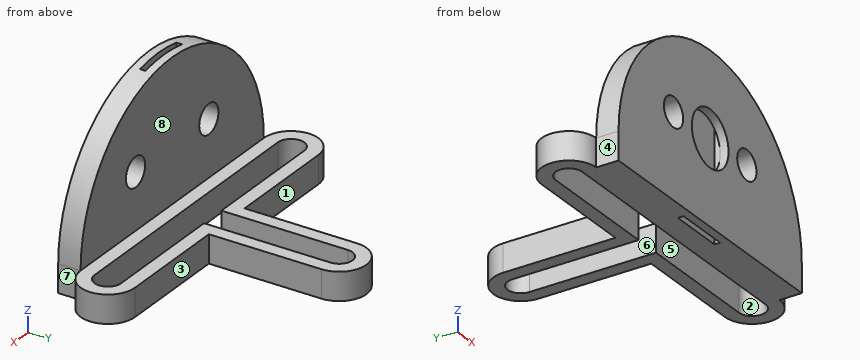
```python
from build123d import *

# Parameters (mm, degrees)
SKETCH1_W           = 100
SKETCH1_H           = 8
BOSS_EXTRUDE1_DEPTH = 10
BOSS_EXTRUDE2_DEPTH = 8
SKETCH3_R           = 5.25
CUT_EXTRUDE1_DEPTH  = 105.404561682
SKETCH4_W           = 20
SKETCH4_H           = 2
CUT_EXTRUDE2_DEPTH  = 104.634574347
SKETCH5_R           = 10
CUT_EXTRUDE3_DEPTH  = 3


with BuildPart() as part:
    # Sketch1 → Boss-Extrude1 (new body)
    # profile 1 of 2: a face of its own
    with BuildSketch(Plane.XY):
        with BuildLine():
            ThreePointArc((-9.75, 50), (0, 59.75), (9.75, 50))
            Line((9.75, 50), (9.75, 9.75))
            Line((9.75, 9.75), (50, 9.75))
            ThreePointArc((50, 9.75), (59.75, 0), (50, -9.75))
            Line((50, -9.75), (-50, -9.75))
            ThreePointArc((-50, -9.75), (-59.75, 0), (-50, 9.75))
            Line((-50, 9.75), (-9.75, 9.75))
            Line((-9.75, 9.75), (-9.75, 50))
        make_face()
        with BuildLine():
            Line((4.75, 4.75), (50, 4.75))
            ThreePointArc((50, 4.75), (54.75, 0), (50, -4.75))
            Line((50, -4.75), (-50, -4.75))
            ThreePointArc((-50, -4.75), (-54.75, 0), (-50, 4.75))
            Line((-50, 4.75), (-4.75, 4.75))
            Line((-4.75, 4.75), (-4.75, 50))
            ThreePointArc((-4.75, 50), (0, 54.75), (4.75, 50))
            Line((4.75, 50), (4.75, 4.75))
        make_face(mode=Mode.SUBTRACT)
    # profile 2 of 2: a face of its own
    with BuildSketch(Plane.XY):
        with Locations((0, -13.75)):
            Rectangle(SKETCH1_W, SKETCH1_H)
    extrude(amount=-BOSS_EXTRUDE1_DEPTH)

    # Sketch2 → Boss-Extrude2 (add)
    with BuildSketch(Plane.XZ.offset(17.75)):
        with BuildLine():
            Line((-50, 0), (50, 0))
            ThreePointArc((50, 0), (0, 50), (-50, 0))
        make_face()
    extrude(amount=-BOSS_EXTRUDE2_DEPTH)

    # Sketch3 → Cut-Extrude1 (cut, through all)
    with BuildSketch(Plane(origin=(0, -9.75, 0), x_dir=(1, 0, 0), z_dir=(0, 1, 0))):
        with Locations(Location((20, -20, 0), (0, 0, 270))):
            Circle(SKETCH3_R)
        with Locations(Location((-20, -20, 0), (0, 0, 270))):
            Circle(SKETCH3_R)
    extrude(amount=-CUT_EXTRUDE1_DEPTH, mode=Mode.SUBTRACT)

    # Sketch4 → Cut-Extrude2 (cut, through all)
    with BuildSketch(Plane(origin=(0, 0, -10), x_dir=(-1, 0, 0), z_dir=(0, 0, -1))):
        with Locations((0, -13.75)):
            Rectangle(SKETCH4_W, SKETCH4_H)
    extrude(amount=-CUT_EXTRUDE2_DEPTH, mode=Mode.SUBTRACT)

    # Sketch5 → Cut-Extrude3 (cut)
    with BuildSketch(Plane.XZ.offset(17.75)):
        with Locations(Location((0, 20, 0), (0, 0, 270))):
            Circle(SKETCH5_R)
    extrude(amount=-CUT_EXTRUDE3_DEPTH, mode=Mode.SUBTRACT)


solid = part.part
```
Check sheet for the modelled part. Datum: model origin and axes. Units: mm. Face numbers are marked on the shaded views. A direction names the side the tool comes from. Round coordinates to 2 decimals unless told otherwise and drop trailing zeros. Write each loop counter-clockwise with the first axis right and the second up, starting at its lowest first coordinate (ties: lowest second). Pieces come first, ordered by that corner, then holes. Notation, with made-up numbers: (55, -37.75) -> (111, -37.75) arc R32 cw to (111, -7.75) -> close; hole circle Ø2 at (45.25, -4). An arc over 180 degrees is marked (long way). One line per question, with ' | ' between items. Start each with the question number.
1. Scan lines: line 1 along Y through (x, z) = (-8.5, -2); line 2 along Y through (x, z) = (-7.5, 45); line 3 along Y through (x, z) = (-35, -4.5). Record each from-to range of solid material in increasing order. Write a range as from..to.
2. Sectioned sample at C-C, the plane z = 16.5. Record the cut outline in (x, y).
3. Sectioned sample at A-A, the plane y = 33. Record the cut outline in (x, z).
4. Sectioned sample at D-D, the plane x = 0. Record the cut outline in (y, z), then the cut area to 3 significant figures.
5. Depth check by flat-ended pin: pin 1 (8 mm diameter, centred on y = 24.5, z = -3.5, fed in from +X); pin 2 (15 mm diameter, centred on x = -15.5, z = 25.5, fed in from +Y); pin 3 (0.6 mm diameter, centred on y = -13.5, z = 8, fed in from +X). Enter the tip coordinate at first touch or a pass-through.
6. Set-up check for the marked faces 1, 2, 3 and 4: record each of +Z, -Z, +X, -X, +Y, -Y from which the full face is reachable in a straight line by a thin tool's end or side.
7. Sectioned sample at B-B, the plane x = 52. Record the cut outline in (y, z).
8. Release check for a two-part mould opening along X. For the marked faces 5, 6, 7 and 8 record: +X half, -X half, draft (parallel to the pull), parting line (faces both ways), or undercut.
Taken from the geometry:
1) line 1: y = -17.75..-14.75, -12.75..-4.75, 4.75..54.78 | line 2: y = -17.75..-14.75, -12.75..-9.75 | line 3: y = -17.75..-4.75, 4.75..9.75
2) outline: (-47.2, -17.75) -> (-23.91, -17.75) -> (-23.91, -9.75) -> (-47.2, -9.75) -> close; (-16.09, -17.75) -> (-9.37, -17.75) -> (-9.37, -14.75) -> (-10, -14.75) -> (-10, -12.75) -> (10, -12.75) -> (10, -14.75) -> (9.37, -14.75) -> (9.37, -17.75) -> (16.09, -17.75) -> (16.09, -9.75) -> (-16.09, -9.75) -> close; (23.91, -17.75) -> (47.2, -17.75) -> (47.2, -9.75) -> (23.91, -9.75) -> close
3) outline: (-9.75, -10) -> (-4.75, -10) -> (-4.75, 0) -> (-9.75, 0) -> close; (4.75, -10) -> (9.75, -10) -> (9.75, 0) -> (4.75, 0) -> close
4) outline: (-17.75, -10) -> (-14.75, -10) -> (-14.75, 10) -> (-17.75, 10) -> close; (-17.75, 30) -> (-14.75, 30) -> (-14.75, 50) -> (-17.75, 50) -> close; (-12.75, -10) -> (-4.75, -10) -> (-4.75, 0) -> (-9.75, 0) -> (-9.75, 50) -> (-12.75, 50) -> close; (54.75, -10) -> (59.75, -10) -> (59.75, 0) -> (54.75, 0) -> close | area: 400 mm^2
5) pin 1: stops at x = 9.75 | pin 2: stops at y = -9.75 | pin 3: stops at x = 49.4
6) face 1: +Z, -Z, -X, +Y | face 2: +Z, -Z | face 3: +Z, -Z, +X, +Y | face 4: +Z, -Z, -X, -Y
7) outline: (-9.54, -10) -> (-4.31, -10) -> (-4.31, 0) -> (-9.54, 0) -> close; (4.31, -10) -> (9.54, -10) -> (9.54, 0) -> (4.31, 0) -> close
8) face 5: undercut | face 6: undercut | face 7: +X half | face 8: draft
